Job drawing, mm, ordinate dimensions from the low corner. One solid piece. Round coordinates to 2 decimals unless told otherwise and drop trailing zeros. Order: outer loops, then holes, each group sorted by start corner. A loop starts at its lowest first (then second) coordinate and runs counter-clockwise, first axis right, second up. Notation, with made-up numbers: (13.5, 24.5) -> (22.5, 24.5) arc R16 ccw to (22.5, 35.5) -> close; hole circle Ø5 at (-14, 55). An arc over 180 degrees is marked (long way). Return JSON: item names as keys, results as strings. Group by question number.
Q1. Cut at B-B (x = 33.5). Write the cut outline in (y, z), then the cut area to 3 significant figures.
Q2. Probe line 1 along X through (y, z) = (12.5, 4); line 2 along X through (y, z) = (15.5, 3.5); line 3 along Y through (x, z) = (10, 3.5). List the from-to ranges inside material, lowest first.
Q3. Cut at C-C (z = 5). Write the cut outline in (x, y), then the cut area to 3 significant figures.
Q4. Flat gauge pins, fed straight in: pin 1 (1 mm diameter, centred on x = 3.5, y = 3.5, fed in from -Z); pin 2 (3 mm diameter, centred on x = 28.5, z = 1.5, fed in from +Y); pin 3 (1.8 mm diameter, centred on x = 3, z = 4, fed in from +Y); pin 4 (1.5 mm diameter, centred on y = 16, z = 2.5, fed in from -X). Where does each tip first touch, or does it go through?
Q5. Mould opens along X. For the marked faces 1 and 2 say: +X half, -X half, draft (parallel to the pull), parting line (faces both ways), or undercut.
Q6. Cut at A-A (y = 11.25). Write the cut outline in (x, z), then the cut area to 3 significant figures.
Q7. Cut at D-D (x = 5.5). Write the cut outline in (y, z).
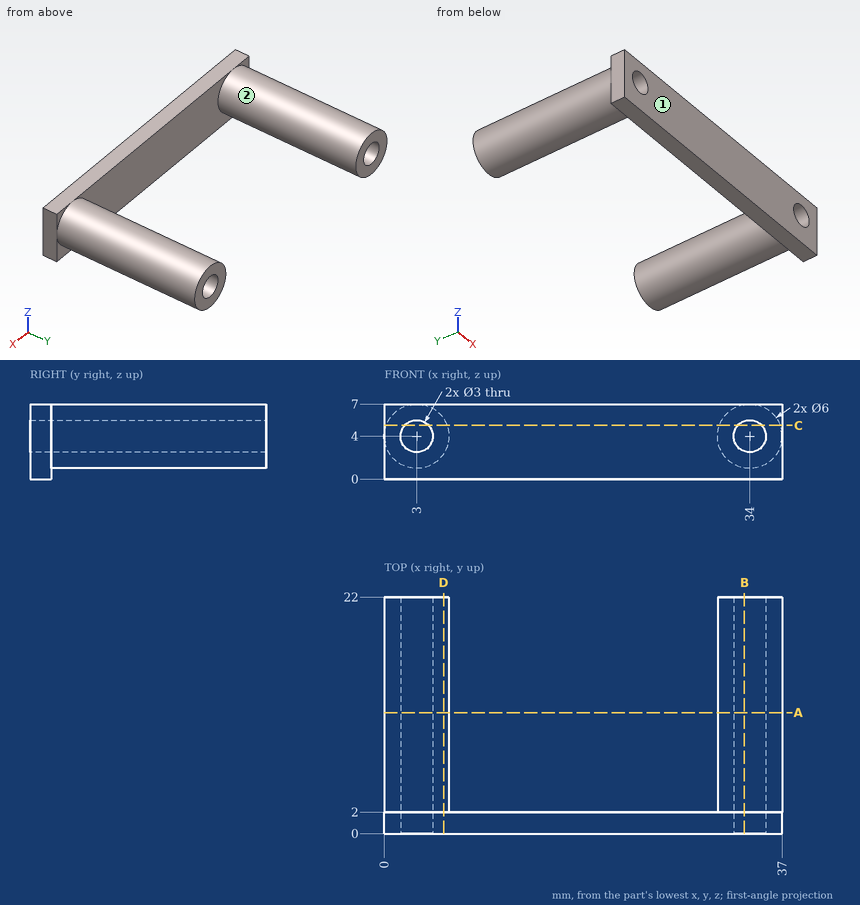
Solution:
{
 "1": {"outline": "(0, 0) -> (2, 0) -> (2, 1.04) -> (22, 1.04) -> (22, 2.59) -> (0, 2.59) -> close; (0, 5.41) -> (22, 5.41) -> (22, 6.96) -> (2, 6.96) -> (2, 7) -> (0, 7) -> close", "area": "70.1 mm²"},
 "2": {"line 1": "x = 0 to 1.5, 4.5 to 6, 31 to 32.5, 35.5 to 37", "line 2": "x = 0.04 to 1.59, 4.41 to 5.96, 31.04 to 32.59, 35.41 to 36.96", "line 3": "y = 0 to 2"},
 "3": {"outline": "(0, 0) -> (1.88, 0) -> (1.88, 22) -> (0.17, 22) -> (0.17, 2) -> (0, 2) -> close; (4.12, 0) -> (32.88, 0) -> (32.88, 22) -> (31.17, 22) -> (31.17, 2) -> (5.83, 2) -> (5.83, 22) -> (4.12, 22) -> close; (35.12, 0) -> (37, 0) -> (37, 2) -> (36.83, 2) -> (36.83, 22) -> (35.12, 22) -> close", "area": "202 mm²"},
 "4": {"pin 1": "stops at z = 1", "pin 2": "stops at y = 2", "pin 3": "passes through", "pin 4": "stops at x = 0.1"},
 "5": {"face 1": "draft", "face 2": "undercut"},
 "6": {"outline": "circle Ø6 at (3, 4); circle Ø6 at (34, 4); hole circle Ø3 at (3, 4); hole circle Ø3 at (34, 4)", "area": "42.4 mm²"},
 "7": {"outline": "(0, 0) -> (2, 0) -> (2, 2.34) -> (22, 2.34) -> (22, 5.66) -> (2, 5.66) -> (2, 7) -> (0, 7) -> close"}
}
